```python
from build123d import *

# Parameters (mm, degrees)
BOSS_EXTRU_1_DEPTH = 50
ESQUISSE2_W        = 18
ESQUISSE2_H        = 50
BOSS_EXTRU_2_DEPTH = 3
CHANFREIN1_SIZE    = 1
CONG_1_R           = 0.5


with BuildPart() as part:
    # Esquisse1 → Boss.-Extru.1 (new body)
    with BuildSketch(Plane.XY):
        Polygon((0, 4.8), (0, 0), (-15, 0), (-15, -3), (3, -3), (3, 8.006659276), (-15.199557032, 6.793355474), (-15, 3.8), align=None)
    extrude(amount=BOSS_EXTRU_1_DEPTH)

    # Esquisse2 → Boss.-Extru.2 (add)
    with BuildSketch(Plane.XZ.offset(3)):
        with Locations((-6, 25)):
            Rectangle(ESQUISSE2_W, ESQUISSE2_H)
        with BuildLine():
            Line((-5.636810707, 25), (-4.842377656, 25.271173743))
            ThreePointArc((-4.842377656, 25.271173743), (-6, 33.1), (-7.157622344, 25.271173743))
            Line((-7.157622344, 25.271173743), (-6.363189293, 25))
            Line((-6.363189293, 25), (-7.157622344, 24.728826257))
            ThreePointArc((-7.157622344, 24.728826257), (-6, 16.9), (-4.842377656, 24.728826257))
            Line((-4.842377656, 24.728826257), (-5.636810707, 25))
        make_face(mode=Mode.SUBTRACT)
    extrude(amount=BOSS_EXTRU_2_DEPTH)

    # Chanfrein1
    chanfrein1_edges = [part.edges().sort_by_distance(p)[0] for p in [
        (-15, 3.8, 25),
        (-15, 0, 25),
    ]]
    chamfer(chanfrein1_edges, length=CHANFREIN1_SIZE)

    # Congé1
    cong_1_edges = [part.edges().sort_by_distance(p)[0] for p in [
        (-6.363189293, -4.5, 25),
        (-5.636810707, -4.5, 25),
    ]]
    fillet(cong_1_edges, radius=CONG_1_R)


solid = part.part
```
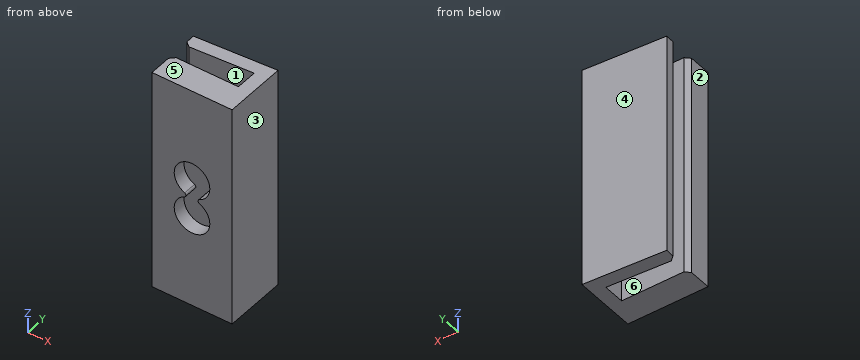
Verification items for the finished model (mm, model axes). Face numbers are marked on the shaded views. A direction names the side the tool comes from. Coordinates: 2 decimals unless noted, no trailing zeros. Write each loop counter-clockwise with the first axis right and the second up, starting at its lowest first coordinate (ties: lowest second). Pieces come first, ordered by that corner, then holes. Notation, with made-up numbers: M 63,-29 L 98,-29 A25 ccw 98,-8 Z; hole C 66,0 d2. An arc over 180 degrees is marked long. Answer as a JSON object with one key per item and string values. Group by question number.
(1) Cross-section at C-C, the plane z = 20.5. Record the cut outline in (x, y).
(2) Material ranges on line 1 (X direction, y = -4.2, z = 29.1); line 2 (X direction, y = 3.25, z = 22.5); line 3 (X direction, y = -1.25, z = 14), recorded low to high.
(3) Tool access check on the marked faces 1, 2 and 3. Record the directions out of +Z, -Z, +X, -X, +Y, -Y that give a thin tool (end or side, any length) a straight path to the whole face; none if there is none.
(4) Cross-section at B-B, the plane z = 29.1. Record the cut outline in (x, y), and give its area (3 significant figures).
(5) Gauge pin test, flat ends, axial feed: pin 1 (1 mm diameter, centred on x = -5.5, y = 2.5, fed in from +Z); pin 2 (1.5 mm diameter, centred on y = -2.5, z = 21, fed in from -X); pin 3 (5 mm diameter, centred on x = -6, z = 20.9, fed in from +Y); pin 4 (7 mm diameter, centred on x = -6, z = 29.1, fed in from -Y). Record the tip position at first contact, or that the pin passes through.
(6) Cross-section at A-A, the plane x = -11.25. Record the cut outline in (y, z).
(7) Cross-section at D-D, the plane x = -6. Record the cut outline in (y, z).
(8) Release check for a two-part mould opening along Y. For the marked faces 4, 5 and 6 record: +Y half, -Y half, draft (parallel to the pull), parting line (faces both ways), or undercut.
Reply:
{
 "1": {"outline": "M -15.2,6.79 L -15.07,4.8 L -14,3.87 L 0,4.8 L 0,0 L -14,0 L -15,-1 L -15,-6 L -9.98,-6 L -9.98,-3 L -2.02,-3 L -2.02,-6 L 3,-6 L 3,8.01 Z"},
 "2": {"line 1": "-15 to -10, -2 to 3", "line 2": "0 to 3", "line 3": "-15 to 3"},
 "3": {"face 1": "+Z, -Z", "face 2": "+Z, -Z, -X, -Y", "face 3": "+Z, -Z, +X, +Y, -Y"},
 "4": {"outline": "M -15.2,6.79 L -15.07,4.8 L -14,3.87 L 0,4.8 L 0,0 L -14,0 L -15,-1 L -15,-6 L -10,-6 L -10,-3 L -2,-3 L -2,-6 L 3,-6 L 3,8.01 Z", "area": "152 mm²"},
 "5": {"pin 1": "through", "pin 2": "x = -15", "pin 3": "y = 7.57", "pin 4": "y = -3"},
 "6": {"outline": "M -6,0 L 0,0 L 0,50 L -6,50 Z; M 4.05,0 L 7.06,0 L 7.06,50 L 4.05,50 Z"},
 "7": {"outline": "M -6,0 L 0,0 L 0,50 L -6,50 L -6,33.1 L -3,33.1 L -3,16.9 L -6,16.9 Z; M 4.4,0 L 7.41,0 L 7.41,50 L 4.4,50 Z"},
 "8": {"face 4": "+Y half", "face 5": "draft", "face 6": "undercut"}
}
